The listing builds one solid part. Answer for the finished solid, in the listing's coordinates (mm). Round coordinates to 2 decimals unless told otherwise and drop trailing zeros. Write each loop counter-clockwise with the first axis right and the second up, starting at its lowest first coordinate (ties: lowest second). Pieces come first, ordered by that corner, then holes. Notation, with made-up numbers: (48.25, 67) - (90.25, 67) arc R15 ccw to (90.25, 92) - close; hole circle Ø3 at (21.25, 64.5). An arc over 180 degrees is marked (long way). Answer in a Markdown table with one row per item.
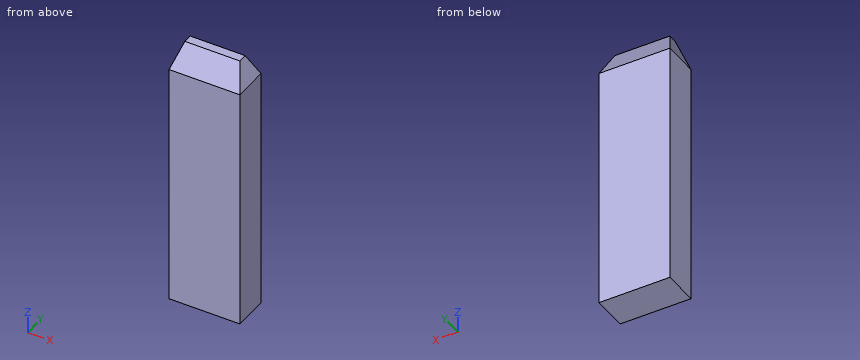
Autodesk Inventor part; units mm, degrees
ref_plane "YZ Plane" through (0, 0, 0) normal (1, 0, 0) x (0, 1, 0)
ref_plane "XZ Plane" through (0, 0, 0) normal (0, 1, 0) x (-1, 0, 0)
ref_plane "XY Plane" through (0, 0, 0) normal (0, 0, 1) x (1, 0, 0)
sketch "Sketch1" plane through (0, 0, 0) normal (0, 1, 0) x (-1, 0, 0)
  line L0 (-2, 0) -> (2, 0)
  line L1 (2, 0) -> (2, 15.35)
  line L2 (2, 15.35) -> (-2, 15.35)
  line L3 (-2, 15.35) -> (-2, 0)
  point P0 (0, 0)
  point P1 (0, 0)
  dimension "d0" = 4
  dimension "d1" = 15.35
extrude "Extrusion1" add sketch "Sketch1" along normal mid plane 2
chamfer "Chamfer1" distance 1.4 distance2 0.45 1 edges at (-2, 0, 15.35) measured on face at (-2, 0.3333, 10.2333)
chamfer "Chamfer2" distance 1.4 distance2 0.45 1 edges at (2, 0, 15.35) measured on face at (2, -0.3333, 10.2333)
chamfer "Chamfer3" distance 1.4 distance2 0.75 1 edges at (0, 1, 15.35) measured on face at (0.6667, 1, 9.3)
chamfer "Chamfer4" distance 1.4 distance2 0.75 1 edges at (0, -1, 15.35) measured on face at (0.6667, -1, 9.3)
properties material "Nickel-Copper Alloy 400"
(1) Find the intervals of material crossed by line 1 (Z direction, x = 0.05, y = -0.4); line 2 (Z direction, x = 0.6, y = 0.8); line 3 (X direction, y = -0.05, z = 14.5), in increasing order.
Checked values:
| item | result |
|---|---|
| line 1 | z = 0 to 15.07 |
| line 2 | z = 0 to 14.32 |
| line 3 | x = -1.82 to 1.82 |
(2) Section B-B (y = 0.7) is taken. Give the vertices of the cut face in (x, z).
Checked values:
| item | result |
|---|---|
| outline | (-2, 0) - (2, 0) - (2, 13.95) - (1.82, 14.51) - (-1.82, 14.51) - (-2, 13.95) - close |
(3) Section C-C (z = 14.25) is taken. Give the vertices of the cut face in (x, y).
Checked values:
| item | result |
|---|---|
| outline | (-1.9, -0.84) - (1.9, -0.84) - (1.9, 0.84) - (-1.9, 0.84) - close |
(4) Section A-A (x = -0.4) is taken. Give the vertices of the cut face in (y, z).
Checked values:
| item | result |
|---|---|
| outline | (-1, 0) - (1, 0) - (1, 13.95) - (0.25, 15.35) - (-0.25, 15.35) - (-1, 13.95) - close |
